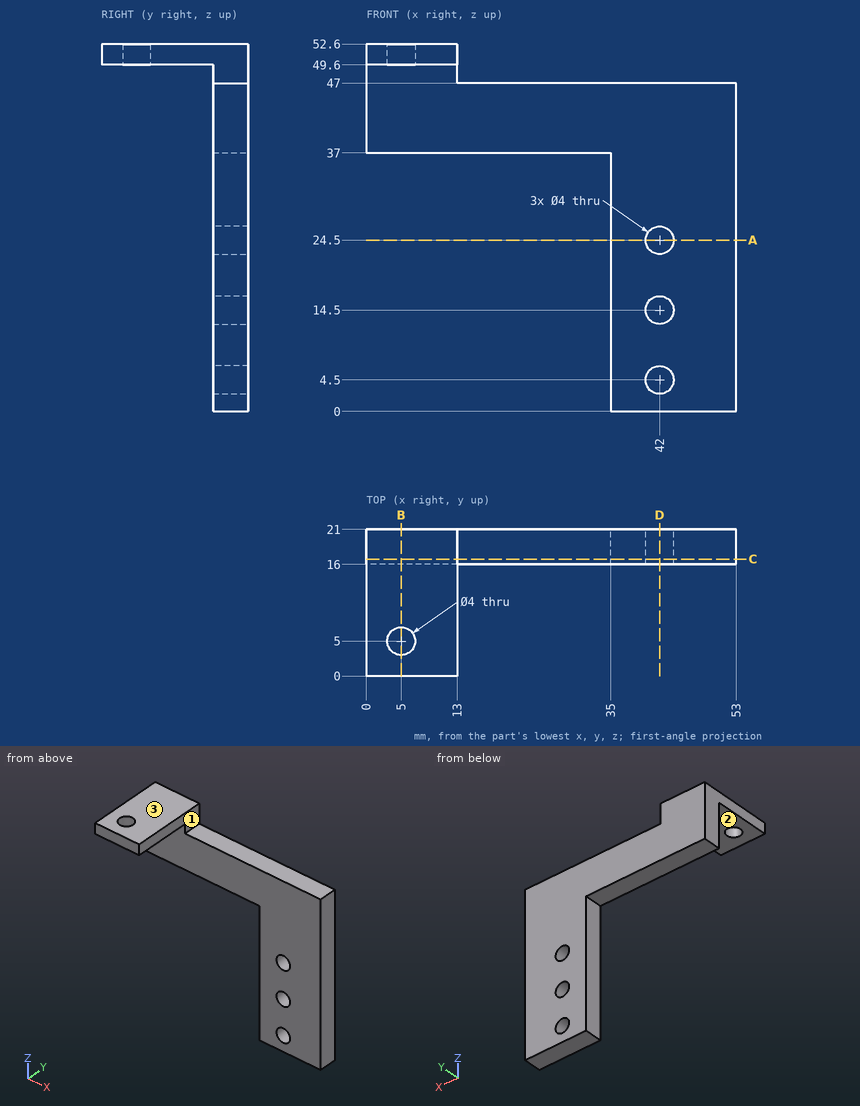
Study the drawing (mm; zero at the part's minimum x, y, z) and answer. A direction names the side the tool comes from. Give positions to 0.01 mm unless a question says otherwise; leave off trailing zeros. Order: outer loops, then holes, each group sorted by start corner. A loop starts at its lowest first (then second) coordinate and runs counter-clockwise, first axis right, second up. Notation, with made-up numbers: (10.25, -19) - (51.25, -19) arc R35 ccw to (51.25, 18) - close; hole circle Ø6 at (-1.5, 87). An arc over 180 degrees is marked (long way). Answer in a Markdown table with one row per item. Add a question column.
Q1. Given P1, Ø5, axis at y = 17, z = 44, coming from the -X side; P2, Ø5.5, axis at x = 20.5, y = 17.5, coming from the -Z side; P3, Ø4, axis at y = 17.5, z = 19, coming from the -X side; P4, Ø4.5, axis at x = 42, z = 24.5, coming from the -Y side, each flat-ended and moving along its own axis, determine where each tip first touches the part or whether it passes through.
Q2. The part is cut by section B-B (x = 5). Determine the outline of the cut face in (y, z).
Q3. The part is cut by section C-C (y = 16.75). Determine the outline of the cut face in (x, z).
Q4. The part is cut by section D-D (x = 42). Determine the outline of the cut face in (y, z), then the cut area to 3 significant figures.
Q5. Which of the six approach directions +Z, -Z, +X, -X, +Y, -Y give full straight-line access (tool end or side, diameter ignored) to the marked faces 1, 2 and 3?
Q6. Find the intervals of material crossed by line 1 along X through (y, z) = (18.45, 4.5); line 2 along Z through (x, y) = (37, 19); line 3 along Z through (x, y) = (40.5, 16.25), in increasing order. Write a range as [from, to].
Q7. The part is cut by section A-A (z = 24.5). Determine the outline of the cut face in (x, y), then the cut area to 3 significant figures.
Determined:
| question | item | result |
|---|---|---|
| 1 | P1 | stops at x = 0 |
| 1 | P2 | stops at z = 37 |
| 1 | P3 | stops at x = 35 |
| 1 | P4 | stops at y = 16 |
| 2 | outline | (0, 49.6) - (3, 49.6) - (3, 52.6) - (0, 52.6) - close; (7, 49.6) - (16, 49.6) - (16, 37) - (21, 37) - (21, 52.6) - (7, 52.6) - close |
| 3 | outline | (0, 37) - (35, 37) - (35, 0) - (53, 0) - (53, 47) - (13, 47) - (13, 52.6) - (0, 52.6) - close; hole circle Ø4 at (42, 4.5); hole circle Ø4 at (42, 14.5); hole circle Ø4 at (42, 24.5) |
| 4 | outline | (16, 0) - (21, 0) - (21, 2.5) - (16, 2.5) - close; (16, 6.5) - (21, 6.5) - (21, 12.5) - (16, 12.5) - close; (16, 16.5) - (21, 16.5) - (21, 22.5) - (16, 22.5) - close; (16, 26.5) - (21, 26.5) - (21, 47) - (16, 47) - close |
| 4 | area | 175 mm² |
| 5 | face 1 | +Z, +X, +Y, -Y |
| 5 | face 2 | -Z, +X, -X, -Y |
| 5 | face 3 | +Z, +X, -X, +Y, -Y |
| 6 | line 1 | x = [35, 40], [44, 53] |
| 6 | line 2 | z = [0, 47] |
| 6 | line 3 | z = [0, 3.18], [5.82, 13.18], [15.82, 23.18], [25.82, 47] |
| 7 | outline | (35, 16) - (40, 16) - (40, 21) - (35, 21) - close; (44, 16) - (53, 16) - (53, 21) - (44, 21) - close |
| 7 | area | 70.0 mm² |
